Can you work these out from the model? Positions are in its coordinate system, mm. A direction names the side the tool comes from. Coordinates: 2 decimals unless noted, no trailing zeros. Loops run counter-clockwise (first coordinate to the right, second up) from the corner with the lowest first, then second, coordinate; pieces in that order, holes last. Notation, with made-up numbers: M 85.25,-36 L 101.25,-36 A20 ccw 101.25,-11 Z; hole C 14.25,82.5 d2. An arc over 180 degrees is marked long. Answer as a JSON object with one key per item and string values. Group by question number.
Item 1: Suppose I cut it at A-A (y = -17). Write out the boundary of the cut face in (x, z).
Item 2: We'd pull the mould along Z, two halves only. Please class faces 1 (the cylindrical face through (41.6, 3.5, -105.3)), 2 (the flat face through (97, -40, -120)): +Z half, -Z half, draft (parallel to the pull), parting line (faces both ways), or undercut.
Item 3: If I drill on line 1 (X direction, y = 1.5, z = -77); line 2 (X direction, y = 5, z = -90); line 3 (Y direction, x = 65, z = -58), over which ranges is the centre line in solid material (lowest first)?
Item 4: Suppose I cut it at B-B (z = -5). Write out the boundary of the cut face in (x, y).
Item 5: Suppose I cut it at C-C (z = -90). Write out the boundary of the cut face in (x, y), then the cut area to 3 significant figures.
Item 6: I'm going to push flat-ended pins straight in: pin 1 Ø3 at (y, z) = (-3.5, -82.5) entering from +X; pin 2 Ø2 at (y, z) = (-1.5, -13.5) entering from +X; pin 3 Ø5 at (x, z) = (51.5, -46.5) entering from -Y; pin 4 Ø2 at (y, z) = (-2.5, -12) entering from -X. Where does each tip first touch, or does it pass through?
Item 7: Suppose I cut it at D-D (z = -41.5). Write out the boundary of the cut face in (x, y).
Item 8: Which directions (+Z, -Z, +X, -X, +Y, -Y) give clear straight access to the entire face, cutting with the end or side of a thin tool? Please do faces 3 (the flat face through (6, -2, -74)), 4 (the flat face through (10, -15, -120)), 5 (the flat face through (3, -2, -77)).
```python
from build123d import *

# Parameters (mm, degrees)
SKETCH2_W           = 100
SKETCH2_H           = 80
BOSS_EXTRUDE1_DEPTH = 10
SKETCH3_W           = 10
SKETCH3_H           = 10
BOSS_EXTRUDE2_DEPTH = 30
SKETCH4_W           = 5
SKETCH4_H           = 10
BOSS_EXTRUDE3_DEPTH = 10
SKETCH5_W           = 6
SKETCH5_H           = 6
BOSS_EXTRUDE4_DEPTH = 4
SKETCH6_R           = 1.5
CUT_EXTRUDE1_DEPTH  = 134.026313187
SKETCH7_W           = 100
SKETCH7_H           = 10
BOSS_EXTRUDE5_DEPTH = 45
SKETCH8_W           = 10
SKETCH8_H           = 10
BOSS_EXTRUDE6_DEPTH = 30
SKETCH9_W           = 5
SKETCH9_H           = 10
BOSS_EXTRUDE7_DEPTH = 10
SKETCH10_R          = 1.5
CUT_EXTRUDE2_DEPTH  = 166
SKETCH11_R          = 1.5
CUT_EXTRUDE3_DEPTH  = 10
CUT_EXTRUDE4_REACH  = 167
SKETCH12_W          = 125
SKETCH12_H          = 3


with BuildPart() as part:
    # Sketch2 → Boss-Extrude1 (new body)
    with BuildSketch(Plane(origin=(0, 0, 0), x_dir=(1, 0, 0), z_dir=(0, 1, 0))):
        with Locations((50, 40)):
            Rectangle(SKETCH2_W, SKETCH2_H)
    extrude(amount=BOSS_EXTRUDE1_DEPTH)

    # Sketch3 → Boss-Extrude2 (add)
    with BuildSketch(Plane.XZ):
        with Locations((95, -5)):
            Rectangle(SKETCH3_W, SKETCH3_H)
        with Locations((5, -5)):
            Rectangle(SKETCH3_W, SKETCH3_H)
    extrude(amount=BOSS_EXTRUDE2_DEPTH)

    # Sketch4 → Boss-Extrude3 (add)
    with BuildSketch(Plane.XZ.offset(30)):
        with Locations((2.5, -5)):
            Rectangle(SKETCH4_W, SKETCH4_H)
        with Locations((97.5, -5)):
            Rectangle(SKETCH4_W, SKETCH4_H)
    extrude(amount=BOSS_EXTRUDE3_DEPTH)

    # Sketch5 → Boss-Extrude4 (add)
    with BuildSketch(Plane.XZ):
        with Locations((6, -13)):
            Rectangle(SKETCH5_W, SKETCH5_H)
        with Locations((95, -13)):
            Rectangle(SKETCH5_W, SKETCH5_H)
        with Locations((95, -77)):
            Rectangle(SKETCH5_W, SKETCH5_H)
        with Locations((6, -77)):
            Rectangle(SKETCH5_W, SKETCH5_H)
    extrude(amount=BOSS_EXTRUDE4_DEPTH)

    # Sketch6 → Cut-Extrude1 (cut, through all)
    with BuildSketch(Plane.XZ.offset(4)):
        with Locations(Location((6, -13, 0), (0, 0, 270))):
            Circle(SKETCH6_R)
        with Locations(Location((95, -13, 0), (0, 0, 270))):
            Circle(SKETCH6_R)
        with Locations(Location((95, -77, 0), (0, 0, 270))):
            Circle(SKETCH6_R)
        with Locations(Location((6, -77, 0), (0, 0, 270))):
            Circle(SKETCH6_R)
    extrude(amount=-CUT_EXTRUDE1_DEPTH, mode=Mode.SUBTRACT)

    # Sketch7 → Boss-Extrude5 (add)
    with BuildSketch(Plane(origin=(0, 0, -80), x_dir=(-1, 0, 0), z_dir=(0, 0, -1))):
        with Locations((-50, 5)):
            Rectangle(SKETCH7_W, SKETCH7_H)
    extrude(amount=BOSS_EXTRUDE5_DEPTH)

    # Sketch8 → Boss-Extrude6 (add)
    with BuildSketch(Plane.XZ):
        with Locations((5, -120)):
            Rectangle(SKETCH8_W, SKETCH8_H)
        with Locations((95, -120)):
            Rectangle(SKETCH8_W, SKETCH8_H)
    extrude(amount=BOSS_EXTRUDE6_DEPTH)

    # Sketch9 → Boss-Extrude7 (add)
    with BuildSketch(Plane.XZ.offset(30)):
        with Locations((2.5, -120)):
            Rectangle(SKETCH9_W, SKETCH9_H)
        with Locations((97.5, -120)):
            Rectangle(SKETCH9_W, SKETCH9_H)
    extrude(amount=BOSS_EXTRUDE7_DEPTH)

    # Sketch10 → Cut-Extrude2 (cut, through all)
    with BuildSketch(Plane.ZY):
        with Locations((-5, -35)):
            Circle(SKETCH10_R)
        with Locations((-120, -35)):
            Circle(SKETCH10_R)
    extrude(amount=-CUT_EXTRUDE2_DEPTH, mode=Mode.SUBTRACT)

    # Sketch11 → Cut-Extrude3 (cut)
    with BuildSketch(Plane.XZ):
        with Locations(Location((4, -106.5, 0), (0, 0, 270))):
            Circle(SKETCH11_R)
        with Locations(Location((4, -90, 0), (0, 0, 270))):
            Circle(SKETCH11_R)
        with Locations(Location((42.5, -106.5, 0), (0, 0, 270))):
            Circle(SKETCH11_R)
        with Locations(Location((42.5, -90, 0), (0, 0, 270))):
            Circle(SKETCH11_R)
    extrude(amount=-CUT_EXTRUDE3_DEPTH, mode=Mode.SUBTRACT)

    # Cut-Extrude4: up to this face of the body (flat: up to its plane)
    cut_extrude4_end = Plane(part.part.faces().sort_by_distance((0, 8.653708798, -62.5))[0])
    # Sketch12 → Cut-Extrude4 (cut, up to the picked face)
    with BuildSketch(Plane(origin=(100, 0, 0), x_dir=(0, 0, -1), z_dir=(1, 0, 0)), mode=Mode.PRIVATE) as cut_extrude4_sk1:
        with Locations((62.5, 8.5)):
            Rectangle(SKETCH12_W, SKETCH12_H)
    cut_extrude4_tool1 = split(extrude(cut_extrude4_sk1.sketch, amount=-CUT_EXTRUDE4_REACH, mode=Mode.PRIVATE), bisect_by=cut_extrude4_end, keep=Keep.BOTH, mode=Mode.PRIVATE)
    add(cut_extrude4_tool1.solids().sort_by(Axis((100, 8.5, -62.5), (-1, 0, 0)))[0], mode=Mode.SUBTRACT)


solid = part.part
```
From the geometry:
{
 "1": {"outline": "M 0,-125 L 10,-125 L 10,-115 L 0,-115 Z; M 0,-10 L 10,-10 L 10,0 L 0,0 Z; M 90,-125 L 100,-125 L 100,-115 L 90,-115 Z; M 90,-10 L 100,-10 L 100,0 L 90,0 Z"},
 "2": {"face 1": "undercut", "face 2": "draft"},
 "3": {"line 1": "0 to 4.5, 7.5 to 93.5, 96.5 to 100", "line 2": "0 to 2.5, 5.5 to 41, 44 to 100", "line 3": "0 to 7"},
 "4": {"outline": "M 0,-40 L 5,-40 L 5,-36.5 L 0,-36.5 Z; M 0,-33.5 L 5,-33.5 L 5,-30 L 10,-30 L 10,0 L 90,0 L 90,-30 L 95,-30 L 95,-33.5 L 100,-33.5 L 100,7 L 0,7 Z; M 95,-40 L 100,-40 L 100,-36.5 L 95,-36.5 Z"},
 "5": {"outline": "M 0,0 L 2.5,0 L 2.5,7 L 0,7 Z; M 5.5,0 L 41,0 L 41,7 L 5.5,7 Z; M 44,0 L 100,0 L 100,7 L 44,7 Z", "area": "658 mm2"},
 "6": {"pin 1": "through", "pin 2": "x = 98", "pin 3": "y = 0", "pin 4": "x = 3"},
 "7": {"outline": "M 0,0 L 100,0 L 100,7 L 0,7 Z"},
 "8": {"face 3": "+X, -X, -Y", "face 4": "+Z, -Z, -Y", "face 5": "-X, -Y"}
}
